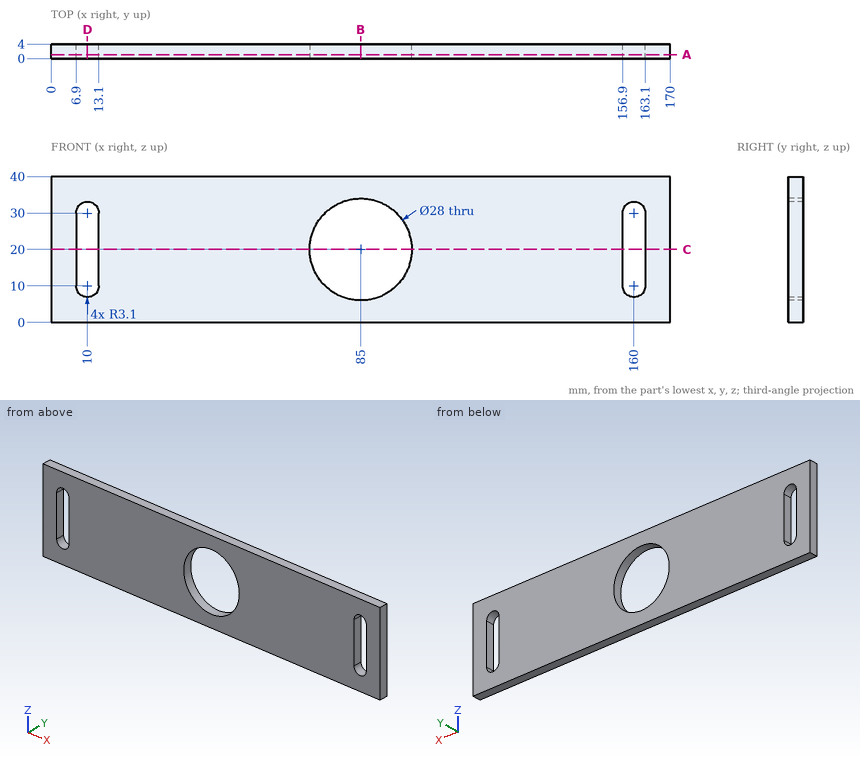
Check sheet for the drawn part. Datum: minimum x, y, z corner. Units: mm. Coordinates: 2 decimals unless noted, no trailing zeros. Write each loop counter-clockwise with the first axis right and the second up, starting at its lowest first coordinate (ties: lowest second). Pieces come first, ordered by that corner, then holes. Notation, with made-up numbers: M 85.25,6 L 123.25,6 A32 cw 123.25,34 Z; hole C 86.5,89 d10. An arc over 180 degrees is marked long. One line per item, written item: value.
Item 1: Section check B-B, the plane x = 85. Record the boundary of the cut face in (y, z), plus the area to 3 significant figures.
Check sheet entries:
outline: M 0,0 L 4,0 L 4,6 L 0,6 Z; M 0,34 L 4,34 L 4,40 L 0,40 Z
area: 48.0 mm^2
Item 2: Section check D-D, the plane x = 10. Record the boundary of the cut face in (y, z).
Check sheet entries:
outline: M 0,0 L 4,0 L 4,6.9 L 0,6.9 Z; M 0,33.1 L 4,33.1 L 4,40 L 0,40 Z
Item 3: Scan lines: line 1 along X through (y, z) = (1.8, 20); line 2 along Z through (x, y) = (85, 1.65); line 3 along X through (y, z) = (3.35, 14.5). Record each from-to range of solid material in increasing order.
Check sheet entries:
line 1: x = 0 to 6.9, 13.1 to 71, 99 to 156.9, 163.1 to 170
line 2: z = 0 to 6, 34 to 40
line 3: x = 0 to 6.9, 13.1 to 72.13, 97.87 to 156.9, 163.1 to 170
Item 4: Section check A-A, the plane y = 1.1. Record the boundary of the cut face in (x, z).
Check sheet entries:
outline: M 0,0 L 170,0 L 170,40 L 0,40 Z; hole M 6.9,10 A3.1 ccw 13.1,10 L 13.1,30 A3.1 ccw 6.9,30 Z; hole C 85,20 d28; hole M 156.9,10 A3.1 ccw 163.1,10 L 163.1,30 A3.1 ccw 156.9,30 Z
Item 5: Section check C-C, the plane z = 20. Record the boundary of the cut face in (x, y), plus the area to 3 significant figures.
Check sheet entries:
outline: M 0,0 L 6.9,0 L 6.9,4 L 0,4 Z; M 13.1,0 L 71,0 L 71,4 L 13.1,4 Z; M 99,0 L 156.9,0 L 156.9,4 L 99,4 Z; M 163.1,0 L 170,0 L 170,4 L 163.1,4 Z
area: 518 mm^2
Item 6: Gauge pin test, flat ends, axial feed: pin 1 Ø3 at (x, z) = (117, 25.5) entering from -Y; pin 2 Ø22.5 at (x, z) = (85, 20) entering from +Y. Record the tip position at first contact, or that the pin passes through.
Check sheet entries:
pin 1: stops at y = 0
pin 2: passes through
